```python
from build123d import *

# Parameters (mm, degrees)
F0_R     = 10
F1_DEPTH = 2
F2_R     = 5.5
F3_DEPTH = 0.3
F4_R     = 4
F5_DEPTH = 3
F6_R     = 0.5


with BuildPart() as f1:
    # F0 (on Top) → F1 (new body)
    with BuildSketch(Plane.XY):
        Circle(F0_R)
    extrude(amount=F1_DEPTH)

    # F2 (on face) → F3 (join)
    with BuildSketch(Plane.XY.offset(2)):
        Circle(F2_R)
    extrude(amount=F3_DEPTH)

    # F4 (on face) → F5 (join)
    with BuildSketch(Plane.XY.offset(2.3)):
        Circle(F4_R)
    extrude(amount=F5_DEPTH)

    # F6
    f6_edges = [f1.edges().sort_by_distance(p)[0] for p in [
        (-4, 0, 5.3),
        (-10, 0, 2),
        (-10, 0, 0),
    ]]
    fillet(f6_edges, radius=F6_R)


solid = f1.part
```
Work out the finished part from the listing and answer in its coordinate system (mm). A direction names the side the tool comes from. Give positions to 0.01 mm unless a question says otherwise; leave off trailing zeros. Loops run counter-clockwise (first coordinate to the right, second up) from the corner with the lowest first, then second, coordinate; pieces in that order, holes last. Notation, with made-up numbers: (54.5, 33) - (64.5, 33) arc R27 ccw to (64.5, 67) - close; hole circle Ø8 at (-13.5, 14.5). An arc over 180 degrees is marked (long way). One line per question, with ' | ' between items.
(1) A tool of negligible diameter and unlimited length cuts with its end or side. For faces 1 (the face through (0, 0, 0)), 2 (the face through (4, -4, 2)), from which of +Z, -Z, +X, -X, +Y, -Y can it reach the whole face along a straight path? Write none if from no direction.
Recorded:
face 1: -Z, +X, -X, +Y, -Y | face 2: +Z
(2) Straight lines are drawn through the part: probe 1 along Z at (x, y) = (7, 0); probe 2 along X at (y, z) = (1, 3.25); probe 3 along X at (y, z) = (-6, 1.65). For each, find the intervals that lie inside material, in ascending order.
Recorded:
probe 1: z = 0 to 2 | probe 2: x = -3.87 to 3.87 | probe 3: x = -7.97 to 7.97
(3) The part is cut by section C-C (z = 2.85). Write down the section's boundary in (x, y).
Recorded:
outline: circle Ø8 at (0, 0)
(4) Each of these flat-tipped pins is pushed along its axis until it touches: pin 1 Ø3 at (y, z) = (-1, 4.5) entering from +X; pin 2 Ø1.5 at (x, z) = (-3.5, 4) entering from +Y; pin 3 Ø1 at (x, z) = (4, 3.5) entering from -Y. Where does it stop, or does it pass through?
Recorded:
pin 1: stops at x = 4 | pin 2: stops at y = 2.9 | pin 3: stops at y = -1.94
(5) The part is cut by section D-D (z = 1.25). Write down the section's boundary in (x, y), then the cut area to 3 significant figures.
Recorded:
outline: circle Ø20 at (0, 0) | area: 314 mm²
(6) The part is cut by section A-A (x = 0). Write down the section's boundary in (y, z).
Recorded:
outline: (-10, 0.5) arc R0.5 ccw to (-9.5, 0) - (9.5, 0) arc R0.5 ccw to (10, 0.5) - (10, 1.5) arc R0.5 ccw to (9.5, 2) - (5.5, 2) - (5.5, 2.3) - (4, 2.3) - (4, 4.8) arc R0.5 ccw to (3.5, 5.3) - (-3.5, 5.3) arc R0.5 ccw to (-4, 4.8) - (-4, 2.3) - (-5.5, 2.3) - (-5.5, 2) - (-9.5, 2) arc R0.5 ccw to (-10, 1.5) - close
